Input: dimensioned drawing with shaded views. Units: mm. Origin: part minimum x, y, z. Round coordinates to 2 decimals unless told otherwise and drop trailing zeros. Write each loop counter-clockwise with the first axis right and the second up, starting at its lowest first coordinate (ties: lowest second). Pieces come first, ordered by that corner, then holes. Notation, with made-up numbers: M 19.5,32.5 L 34.5,32.5 A30 cw 34.5,62.5 Z; hole C 51.25,81 d10. An arc over 180 degrees is marked long. Answer as CSV lines item,"result". Start each with the question number.
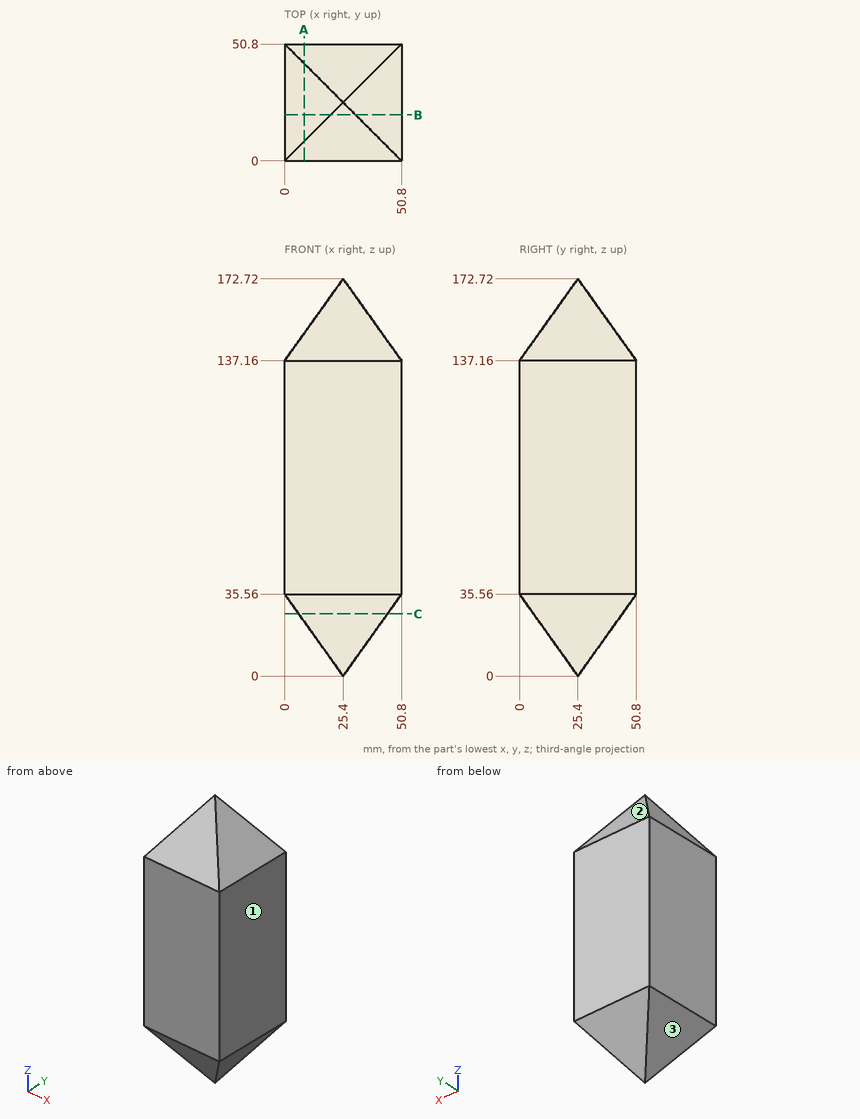
Item 1: Draft query along Z for the marked faces 1, 2 and 3. Return one class per face: +Z half, -Z half, draft (parallel to the pull), parting line (faces both ways), or undercut.
Item 2: Cut plane C-C, the plane z = 27. Return loops of the section in (x, y).
Item 3: Pin query (flat end, axial travel): pin 1 Ø10 at (x, y) = (36, 16.5) entering from +Z; pin 2 Ø12 at (x, y) = (16.5, 32.5) entering from -Z; pin 3 Ø10 at (x, y) = (43.5, 11) entering from +Z. Return the tip coordinate at first contact, or that it passes through.
Item 4: Line query: line 1 (Y direction, x = 8.5, z = 146); line 2 (Z direction, x = 43.5, y = 22); line 3 (Y direction, x = 36.5, z = 141.5). Output: solid intervals per line, ascending. Write a range as [from, to].
Item 5: Cut plane B-B, the plane y = 20. Return loops of the section in (x, z), plus the area to 3 significant figures.
Item 6: Cut plane A-A, the plane x = 8.5. Return loops of the section in (y, z).
Results list:
1,face 1,"draft"
1,face 2,"+Z half"
1,face 3,"-Z half"
2,outline,"M 6.11,6.11 L 44.69,6.11 L 44.69,44.69 L 6.11,44.69 Z"
3,pin 1,"z = 163.87"
3,pin 2,"z = 5.4"
3,pin 3,"z = 154.19"
4,line 1,"[6.31, 44.49]"
4,line 2,"[25.34, 147.38]"
4,line 3,"[3.1, 47.7]"
5,outline,"M 0,35.56 L 20,7.56 L 30.8,7.56 L 50.8,35.56 L 50.8,137.16 L 30.8,165.16 L 20,165.16 L 0,137.16 Z"
5,area,"6,890 mm²"
6,outline,"M 0,35.56 L 8.5,23.66 L 42.3,23.66 L 50.8,35.56 L 50.8,137.16 L 42.3,149.06 L 8.5,149.06 L 0,137.16 Z"
